```python
from build123d import *

# Parameters (mm, degrees)
F1_DEPTH      = 125
F1_DEPTH_BACK = 125
F6_DEPTH      = 5.0009999999
F7_DEPTH      = 5.0010000001
F8_DEPTH      = 2
F9_DEPTH      = 2
F10_DEPTH     = 2
F11_DEPTH     = 2
F12_W         = 30
F12_H         = 40
F13_DEPTH     = 35.001
F14_R         = 17.49999


# Not quite as in the source:
# - a fillet or chamfer is up to 0.001 mm smaller than in the source, because OpenCascade refuses the exact size


with BuildPart() as f1:
    # F0 (on Front) → F1 (new body, two sides)
    with BuildSketch(Plane.XZ) as f1_sk:
        Polygon((-20, -17.5), (20, -17.5), (20, 17.5), (15, 17.5), (15, -11.25), (-15, -11.25), (-15, 17.5), (-20, 17.5), align=None)
    extrude(amount=F1_DEPTH)
    extrude(f1_sk.sketch, amount=-F1_DEPTH_BACK)

    # F3 (on face) → F6 (cut, through all)
    with BuildSketch(Plane(origin=(15.0000000001, 0, 0), x_dir=(0, -1, 0), z_dir=(-1, 0, 0))):
        with BuildLine():
            Line((107.5, 4.9999999999), (0, 4.9999999999))
            Line((0, 4.9999999999), (-107.5, 4.9999999999))
            ThreePointArc((-107.5, 4.9999999999), (-112.5, -2e-10), (-107.5, -5.0000000004))
            Line((-107.5, -5.0000000004), (0, -5.0000000004))
            Line((0, -5.0000000004), (107.5, -5.0000000004))
            ThreePointArc((107.5, -5.0000000004), (112.5000000001, -2e-10), (107.5, 4.9999999999))
        make_face()
    extrude(amount=-F6_DEPTH, mode=Mode.SUBTRACT)

    # F2 (on face) → F7 (cut, through all)
    with BuildSketch(Plane.YZ.offset(-14.9999999999)):
        with BuildLine():
            Line((107.5, 5), (0, 5))
            Line((0, 5), (-107.5, 5))
            ThreePointArc((-107.5, 5), (-112.5, 0), (-107.5, -5))
            Line((-107.5, -5), (0, -5))
            Line((0, -5), (107.5, -5))
            ThreePointArc((107.5, -5), (112.5, 0), (107.5, 5))
        make_face()
    extrude(amount=-F7_DEPTH, mode=Mode.SUBTRACT)

    # F3 (on face) → F8 (cut)
    with BuildSketch(Plane(origin=(15.0000000001, 0, 0), x_dir=(0, -1, 0), z_dir=(-1, 0, 0))):
        with BuildLine():
            Line((107.5, 11.25), (0, 11.25))
            Line((0, 11.25), (-107.5, 11.25))
            ThreePointArc((-107.5, 11.25), (-118.7500000002, -2e-10), (-107.5, -11.2500000005))
            Line((-107.5, -11.2500000005), (0, -11.2500000005))
            Line((0, -11.2500000005), (107.5, -11.2500000005))
            ThreePointArc((107.5, -11.2500000005), (118.7500000002, -2e-10), (107.5, 11.25))
        make_face()
        with BuildLine():
            Line((-107.5, 4.9999999999), (0, 4.9999999999))
            Line((0, 4.9999999999), (107.5, 4.9999999999))
            ThreePointArc((107.5, 4.9999999999), (112.5000000001, -2e-10), (107.5, -5.0000000004))
            Line((107.5, -5.0000000004), (0, -5.0000000004))
            Line((0, -5.0000000004), (-107.5, -5.0000000004))
            ThreePointArc((-107.5, -5.0000000004), (-112.5, -2e-10), (-107.5, 4.9999999999))
        make_face(mode=Mode.SUBTRACT)
    extrude(amount=-F8_DEPTH, mode=Mode.SUBTRACT)

    # F2 (on face) → F9 (cut)
    with BuildSketch(Plane.YZ.offset(-14.9999999999)):
        with BuildLine():
            Line((107.5, 11.25), (0, 11.25))
            Line((0, 11.25), (-107.5, 11.25))
            ThreePointArc((-107.5, 11.25), (-118.75, 0), (-107.5, -11.25))
            Line((-107.5, -11.25), (0, -11.25))
            Line((0, -11.25), (107.5, -11.25))
            ThreePointArc((107.5, -11.25), (118.75, 0), (107.5, 11.25))
        make_face()
        with BuildLine():
            Line((-107.5, 5), (0, 5))
            Line((0, 5), (107.5, 5))
            ThreePointArc((107.5, 5), (112.5, 0), (107.5, -5))
            Line((107.5, -5), (0, -5))
            Line((0, -5), (-107.5, -5))
            ThreePointArc((-107.5, -5), (-112.5, 0), (-107.5, 5))
        make_face(mode=Mode.SUBTRACT)
    extrude(amount=-F9_DEPTH, mode=Mode.SUBTRACT)

    # F4 (on face) → F10 (cut)
    with BuildSketch(Plane(origin=(-20, 0, 1e-10), x_dir=(0, -1, 0), z_dir=(-1, 0, 0))):
        with BuildLine():
            Line((107.5, 11.25), (0, 11.25))
            Line((0, 11.25), (-107.5, 11.25))
            ThreePointArc((-107.5, 11.25), (-118.75, 0), (-107.5, -11.25))
            Line((-107.5, -11.25), (0, -11.25))
            Line((0, -11.25), (107.5, -11.25))
            ThreePointArc((107.5, -11.25), (118.75, 0), (107.5, 11.25))
        make_face()
        with BuildLine():
            Line((-107.5, 5), (0, 5))
            Line((0, 5), (107.5, 5))
            ThreePointArc((107.5, 5), (112.5, 0), (107.5, -5))
            Line((107.5, -5), (0, -5))
            Line((0, -5), (-107.5, -5))
            ThreePointArc((-107.5, -5), (-112.5, 0), (-107.5, 5))
        make_face(mode=Mode.SUBTRACT)
    extrude(amount=-F10_DEPTH, mode=Mode.SUBTRACT)

    # F5 (on face) → F11 (cut)
    with BuildSketch(Plane.YZ.offset(20)):
        with BuildLine():
            Line((107.5, 11.25), (0, 11.25))
            Line((0, 11.25), (-107.5, 11.25))
            ThreePointArc((-107.5, 11.25), (-118.75, 0), (-107.5, -11.25))
            Line((-107.5, -11.25), (0, -11.25))
            Line((0, -11.25), (107.5, -11.25))
            ThreePointArc((107.5, -11.25), (118.75, 0), (107.5, 11.25))
        make_face()
        with BuildLine():
            Line((-107.5, 5), (0, 5))
            Line((0, 5), (107.5, 5))
            ThreePointArc((107.5, 5), (112.5, 0), (107.5, -5))
            Line((107.5, -5), (0, -5))
            Line((0, -5), (-107.5, -5))
            ThreePointArc((-107.5, -5), (-112.5, 0), (-107.5, 5))
        make_face(mode=Mode.SUBTRACT)
    extrude(amount=-F11_DEPTH, mode=Mode.SUBTRACT)

    # F12 (on face) → F13 (cut, through all)
    with BuildSketch(Plane(origin=(0, 0, -17.5), x_dir=(1, 0, 0), z_dir=(0, 0, -1))):
        with Locations((-2e-10, -105)):
            Rectangle(F12_W, F12_H)
        with Locations((-2e-10, 105)):
            Rectangle(F12_W, F12_H)
    extrude(amount=-F13_DEPTH, mode=Mode.SUBTRACT)

    # F14 (radius 17.5 in the source; OpenCascade refuses exactly that, so slightly less here)
    f14_edges = [f1.edges().sort_by_distance(p)[0] for p in [
        (17.5, 125, 17.5),
        (17.5, 125, -17.5),
        (-17.5, 125, -17.5),
        (-17.5, 125, 17.5),
        (-17.5, -125, -17.5),
        (-17.5, -125, 17.5),
        (17.5, -125, 17.5),
        (17.5, -125, -17.5),
    ]]
    fillet(f14_edges, radius=F14_R)


solid = f1.part
```
For this review, take the finished solid that the model builds, in its own axes (mm). A direction names the side the tool comes from. Round coordinates to 2 decimals unless told otherwise and drop trailing zeros. Order: outer loops, then holes, each group sorted by start corner. A loop starts at its lowest first (then second) coordinate and runs counter-clockwise, first axis right, second up.
Q1. Mouldability with a two-part tool opening along Z and no side actions: class faces 1 (the cylindrical face through (17.46, 120.01, 12.24)), 2 (the flat face through (17, 1.7, 5.2)), 3 (the cylindrical face through (15.986, -118.747, -0.247)), 4 (the cylindrical face through (-17.47, 119.74, -12.51)) as pulls with the +Z half, pulls with the -Z half, needs draft (parallel to the pull), parting line crosses it, or undercut.
Findings below:
face 1: pulls with the +Z half
face 2: undercut
face 3: undercut
face 4: pulls with the -Z half
Q2. Wall thickness on line 1 (X direction, y = -89, z = -7.5); line 2 (Y direction, x = -16.5, z = 0.5); line 3 (Z direction, x = 18.5, y = -101): over which ranges is each line inside the solid? List them lowest first.
Findings below:
line 1: x = -18 to -17, 17 to 18
line 2: y = -124.99 to -118.74, 118.74 to 124.99
line 3: z = -17.5 to -11.25, 11.25 to 17.5
Q3. Insertion check: P1, Ø6, axis at y = -59, z = -5, coming from the +X side; P2, Ø3, axis at x = 3.5, z = -13.5, coming from the +Y side; P3, Ø5, axis at y = 41.5, z = 7, coming from the -X side. Each pin has a flat end and moves straight along its axis. Give the tip position at first contact, or say it passes through.
Findings below:
P1: stops at x = 18
P2: stops at y = 85
P3: stops at x = -18
Q4. We need section A-A, the plane y = 10.5. Give the boundary of the cut face in (x, z), plus the area to 4 significant figures.
Findings below:
outline: (-20, -17.5) - (20, -17.5) - (20, -11.25) - (18, -11.25) - (18, -5) - (17, -5) - (17, -11.25) - (-17, -11.25) - (-17, -5) - (-18, -5) - (-18, -11.25) - (-20, -11.25) - close; (-20, 11.25) - (-18, 11.25) - (-18, 5) - (-17, 5) - (-17, 11.25) - (-15, 11.25) - (-15, 17.5) - (-20, 17.5) - close; (15, 11.25) - (17, 11.25) - (17, 5) - (18, 5) - (18, 11.25) - (20, 11.25) - (20, 17.5) - (15, 17.5) - close
area: 337.5 mm2
Q5. We need section C-C, the plane x = 0.5. Give the boundary of the cut face in (y, z), plus the area to 3 significant figures.
Findings below:
outline: (-85, -17.5) - (85, -17.5) - (85, -11.25) - (-85, -11.25) - close
area: 1,060 mm2
Q6. Machinability: for faces 5 (the cylindrical face through (19.014, 118.747, -0.247)), 6 (the cylindrical face through (-15.986, -118.747, 0.247)), 7 (the flat face through (0, -85, -14)), which of the approach directions +Z, -Z, +X, -X, +Y, -Y give a long, thin tool a straight path to every point of the face, cutting with its end or side? Answer none if there is none.
Findings below:
face 5: +X
face 6: none
face 7: +Z, -Z, -Y
Q7. We need section B-B, the plane z = 15. Give the boundary of the cut face in (x, y), plus the area to 3 significant figures.
Findings below:
outline: (-20, -116.51) - (-15, -116.51) - (-15, 116.51) - (-20, 116.51) - close; (15, -116.51) - (20, -116.51) - (20, 116.51) - (15, 116.51) - close
area: 2,330 mm2
